Drawing for the job (mm, zero at the part's lowest x, y, z). Give positions to 0.01 mm unless a question says otherwise; leave off trailing zeros. Loops run counter-clockwise (first coordinate to the right, second up) from the corner with the lowest first, then second, coordinate; pieces in that order, holes last. Notation, with made-up numbers: (65.5, 35) -> (104.5, 35) arc R13 ccw to (104.5, 43) -> close; hole circle Ø5 at (-35.75, 19.5). An arc over 180 degrees is marked (long way). Use CSV: the item, a comma, the result in double quotes. Start each with the question number.
(1) Drill centre lines: probe 1 along X at (y, z) = (81.5, 6.25); probe 2 along Y at (x, z) = (286.5, 1.75). Where is each one in solid material? Low to high.
(2) Cut at A-A on z = 15. Write the cut outline in (x, y).
(3) Pull direction Z, two halves, no side cores. Call the marked faces 1 and 2: pulls with the +Z half, pulls with the -Z half, needs draft (parallel to the pull), parting line crosses it, or undercut.
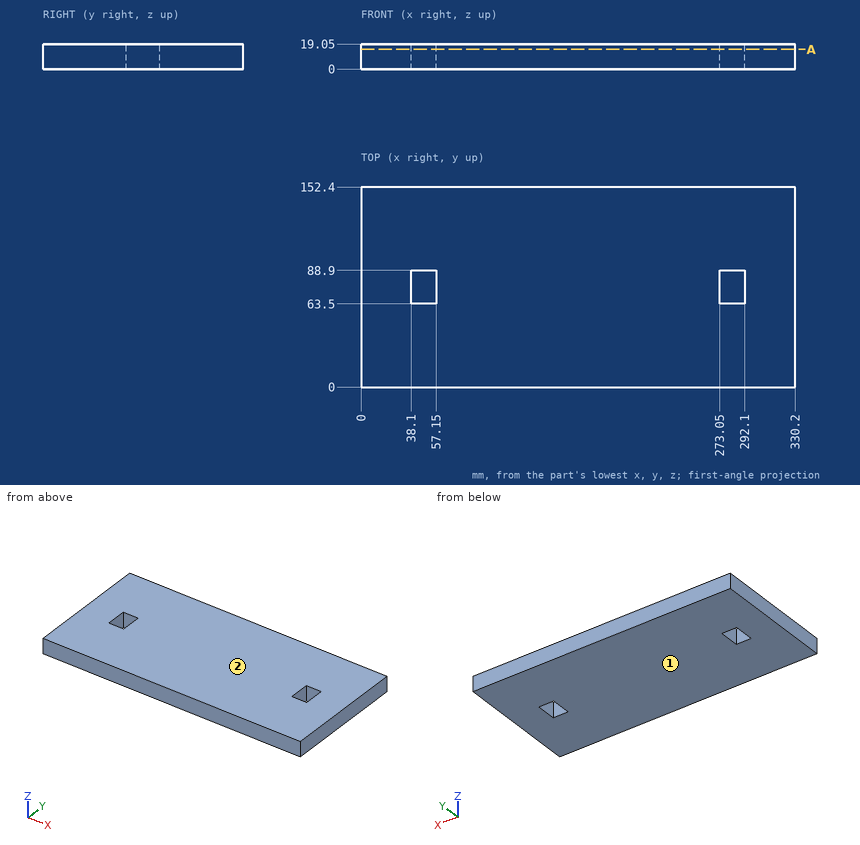
Check result:
1,probe 1,"0 to 38.1, 57.15 to 273.05, 292.1 to 330.2"
1,probe 2,"0 to 63.5, 88.9 to 152.4"
2,outline,"(0, 0) -> (330.2, 0) -> (330.2, 152.4) -> (0, 152.4) -> close; hole (38.1, 63.5) -> (57.15, 63.5) -> (57.15, 88.9) -> (38.1, 88.9) -> close; hole (273.05, 63.5) -> (292.1, 63.5) -> (292.1, 88.9) -> (273.05, 88.9) -> close"
3,face 1,"pulls with the -Z half"
3,face 2,"pulls with the +Z half"
